from build123d import *

# Parameters (mm, degrees)
SKETCH1_R             = 3
BOSS_EXTRUDE2_DEPTH   = 12.7
CROQUIS3_R            = 2
CORTAR_EXTRUIR2_DEPTH = 25


with BuildPart() as part:
    # Sketch1 → Boss-Extrude2 (new body)
    with BuildSketch(Plane(origin=(0, 0, 0), x_dir=(0, 0, -1), z_dir=(1, 0, 0))):
        with BuildLine():
            Line((49.204101374, 10.956842444), (15.890879059, 47.035174964))
            ThreePointArc((15.890879059, 47.035174964), (14.889789553, 47.748228965), (13.686777685, 48))
            Line((13.686777685, 48), (1, 48))
            ThreePointArc((1, 48), (-11.499928284, 35.457657454), (1.084684606, 23.000286863))
            ThreePointArc((1.084684606, 23.000286863), (18.871740524, 15.738310099), (26.254053819, -1.999139412))
            Line((26.254053819, -1.999139412), (64, -1.999139412))
            Line((64, -1.999139412), (64, 2.000860588))
            ThreePointArc((64, 2.000860588), (63.414213562, 3.41507415), (62, 4.000860588))
            Line((62, 4.000860588), (50, 4.000860588))
            Line((50, 4.000860588), (50, 8.921667481))
            ThreePointArc((50, 8.921667481), (49.793949187, 10.014300969), (49.204101374, 10.956842444))
        make_face()
        with Locations((1, 35.5)):
            Circle(SKETCH1_R, mode=Mode.SUBTRACT)
        with BuildLine():
            Line((42.469400916, 13.828321623), (17.083800106, 41.321013221))
            ThreePointArc((17.083800106, 41.321013221), (14.885976864, 41.826862703), (13.61439919, 39.964229912))
            Line((13.61439919, 39.964229912), (13.61439919, 25.251581588))
            ThreePointArc((13.61439919, 25.251581588), (13.901973758, 24.218334695), (14.681998331, 23.482223332))
            ThreePointArc((14.681998331, 23.482223332), (23.753909667, 15.98324163), (29.068629616, 5.481429706))
            ThreePointArc((29.068629616, 5.481429706), (29.78321361, 4.413589067), (31, 4.000860588))
            Line((31, 4.000860588), (41, 4.000860588))
            ThreePointArc((41, 4.000860588), (42.414213562, 4.586647025), (43, 6.000860588))
            Line((43, 6.000860588), (43, 12.471538314))
            ThreePointArc((43, 12.471538314), (42.862632792, 13.199960639), (42.469400916, 13.828321623))
        make_face(mode=Mode.SUBTRACT)
    extrude(amount=BOSS_EXTRUDE2_DEPTH)

    # Croquis3 → Cortar-Extruir2 (cut)
    with BuildSketch(Plane(origin=(0, 4.000860588, 0), x_dir=(1, 0, 0), z_dir=(0, 1, 0))):
        with Locations(Location((6.35, 56, 0), (0, 0, 270))):
            Circle(CROQUIS3_R)
        with Locations(Location((6.35, 36, 0), (0, 0, 270))):
            Circle(CROQUIS3_R)
    extrude(amount=-CORTAR_EXTRUIR2_DEPTH, mode=Mode.SUBTRACT)


solid = part.part
The model under review builds one solid part; all positions refer to its coordinate system, in mm. A direction names the side the tool comes from. Round coordinates to 2 decimals unless told otherwise and drop trailing zeros. Write each loop counter-clockwise with the first axis right and the second up, starting at its lowest first coordinate (ties: lowest second). Pieces come first, ordered by that corner, then holes. Notation, with made-up numbers: M -24.5,46.5 L 27.5,46.5 A16 cw 27.5,63.5 Z; hole C 72.25,-32 d8. An arc over 180 degrees is marked long. Answer as CSV lines item,"result". Start each with the question number.
Q1. Consider section A-A, the plane z = -56. Give the boundary of the cut face in (x, y).
Q2. The part is to be moulded in two halves that separate along X. For faces 1 (the face through (5.584, 1.043, -54.153)), 2 (the face through (12.7, 23, -15)), 3 (the face through (6.26, 4.57, -42.4)), 4 (the face through (5.584, 1.043, -34.153)), say which applies: +X half, -X half, draft (parallel to the pull), parting line (faces both ways), or undercut.
Q3. Wall thickness on line 1 along X through (y, z) = (0, -56); line 2 along Z through (x, y) = (7, 34.5); line 3 along Y through (x, z) = (5, 0): over which ranges is each line inside the solid? List them lowest first.
Q4. Consider section C-C, the plane x = 1.5. Give the boundary of the cut face in (y, z).
Q5. Tool access review of faces 5 (the face through (6.261, 27.382, -29.954)), 6 (the face through (6, 4.001, -59)), 7 (the face through (6, 0, -64)): name each direction out of +Z, -Z, +X, -X, +Y, -Y from which nothing blocks a thin tool from reaching the whole face with its end or side.
Q6. Clearance check with flat-ended pins moving along their axes: P1, Ø3.5, axis at y = 35.5, z = -1, coming from the -X side; P2, Ø6, axis at x = 1.5, z = -55.5, coming from the +Y side; P3, Ø1, axis at x = 9.5, z = -14.5, coming from the +Y side; P4, Ø4.5, axis at x = 6.35, z = -36, coming from the +Y side. State where each tip first meets the part, or that it passes through.
Q7. Consider section D-D, the plane y = 21. Give the boundary of the cut face in (x, z), then the cut area to 3 significant figures.
Q8. Consider section B-B, the plane y = 35.5. Give the boundary of the cut face in (x, z).
Result set:
1,outline,"M 0,-2 L 4.35,-2 L 4.35,4 L 0,4 Z; M 8.35,-2 L 12.7,-2 L 12.7,4 L 8.35,4 Z"
2,face 1,"undercut"
2,face 2,"+X half"
2,face 3,"draft"
2,face 4,"undercut"
3,line 1,"x = 0 to 4.35, 8.35 to 12.7"
3,line 2,"z = -27.47 to -23.38, -13.61 to -3.83, 1.83 to 11.46"
3,line 3,"y = 23.04 to 32.67, 38.33 to 47.96"
4,outline,"M -2,-64 L 2,-64 A2 ccw 4,-62 L 4,-50 L 8.92,-50 A3 ccw 10.96,-49.2 L 47.04,-15.89 A3 ccw 48,-13.69 L 48,-1 A12.5 ccw long 23,-1.08 A25 cw -2,-26.25 Z; hole M 4,-41 A2 ccw 6,-43 L 12.47,-43 A2 ccw 13.83,-42.47 L 41.32,-17.08 A2 ccw 39.96,-13.61 L 25.25,-13.61 A2 ccw 23.48,-14.68 A28.8 cw 5.48,-29.07 A2 ccw 4,-31 Z; hole C 35.5,-1 d6"
5,face 5,"+X, -X"
5,face 6,"-Z, +X, -X, +Y"
5,face 7,"-Z, +X, -X, +Y, -Y"
6,P1,"passes through"
6,P2,"stops at y = 4"
6,P3,"stops at y = 47.98"
6,P4,"stops at y = 27.69"
7,outline,"M 0,-39.93 L 12.7,-39.93 L 12.7,-35.85 L 0,-35.85 Z; M 0,-18.59 L 12.7,-18.59 L 12.7,-11.05 L 0,-11.05 Z"
7,area,"148 mm²"
8,outline,"M 0,-26.54 L 12.7,-26.54 L 12.7,-22.46 L 0,-22.46 Z; M 0,-13.61 L 12.7,-13.61 L 12.7,-4 L 0,-4 Z; M 0,2 L 12.7,2 L 12.7,11.5 L 0,11.5 Z"
